Can you work these out from the model? Positions are in its coordinate system, mm. Face numbers are marked on the shaded views. Give positions to 0.01 mm unless a question says otherwise; leave off trailing zeros. Loops run counter-clockwise (first coordinate to the right, second up) from the corner with the lowest first, then second, coordinate; pieces in that order, holes last. Notation, with made-up numbers: (52, -2) -> (86, -2) arc R23 ccw to (86, 17) -> close; hole circle Ø9 at (-27, 9.5). An arc over 180 degrees is marked (long way). Return JSON: item names as keys, results as strings. Group by question number.
Q1. Suppose I cut it at C-C, the plane y = 31. Please give me the cut outline in (x, z).
Q2. I need wall thicknesses on line 1 along Z through (x, y) = (11, 20.5); line 2 along Z through (x, y) = (-0.5, 27); line 3 along X through (y, z) = (44.5, 36). Which ranges of each line are inside material? Lowest first, please. Write a range as [from, to].
Q3. Suppose I cut it at B-B, the plane x = 5. Count the separate pieces of the cut face and the enclosed holes in it, and give its area (3 significant figures).
Q4. Thinking about a two-plate mould opening in X: for the marked faces 1, 2, 3 and 4, which applies, pulls with the +X half, pulls with the -X half, needs draft (parallel to the pull), parting line crosses it, or undercut?
Q5. Suppose I cut it at A-A, the plane y = 4. Please give me the cut outline in (x, z).
```python
from build123d import *

# Parameters (mm, degrees)
SKETCH2_W           = 54.8
SKETCH2_H           = 95
BOSS_EXTRUDE1_DEPTH = 50.8
SKETCH3_R           = 19.05
CUT_EXTRUDE1_DEPTH  = 5
SKETCH4_R           = 14.435817204
SKETCH4_166_R       = 14.435817204


with BuildPart() as part:
    # Sketch2 → Boss-Extrude1 (new body)
    with BuildSketch(Plane(origin=(0, 0, 0), x_dir=(1, 0, 0), z_dir=(0, 1, 0))):
        with Locations((0, -0.795454545)):
            Rectangle(SKETCH2_W, SKETCH2_H)
    extrude(amount=BOSS_EXTRUDE1_DEPTH)

    # Sketch3 → Cut-Extrude1 (cut)
    with BuildSketch(Plane.XZ):
        with Locations(Location((-0.029477, 26.254895545, 0), (0, 0, 270))):
            Circle(SKETCH3_R)
        with Locations(Location((-0.029477, -24.545104455, 0), (0, 0, 90))):
            Circle(SKETCH3_R)
    extrude(amount=-CUT_EXTRUDE1_DEPTH, mode=Mode.SUBTRACT)

    # Sketch4 → section 0 of cut_loft1
    with BuildSketch(Plane(origin=(0, 50.8, 0), x_dir=(1, 0, 0), z_dir=(0, 1, 0)), mode=Mode.PRIVATE) as cut_loft1_s0:
        with Locations((-0.029477, 24.545104455)):
            Circle(SKETCH4_R)
    # loft up to a face of the part (cut_loft1)
    loft([cut_loft1_s0.sketch, Face(Wire([part.edges().sort_by_distance((-13.916329352, 5, -37.585726822))[0]]))], mode=Mode.SUBTRACT)

    # Sketch4<166> → section 0 of cut_loft2
    with BuildSketch(Plane(origin=(0, 50.8, 0), x_dir=(1, 0, 0), z_dir=(0, 1, 0)), mode=Mode.PRIVATE) as cut_loft2_s0:
        with Locations((-0.029477, -26.254895545)):
            Circle(SKETCH4_166_R)
    # loft up to a face of the part (cut_loft2)
    loft([cut_loft2_s0.sketch, Face(Wire([part.edges().sort_by_distance((13.857375352, 5, 39.295517913))[0]]))], mode=Mode.SUBTRACT)


solid = part.part
```
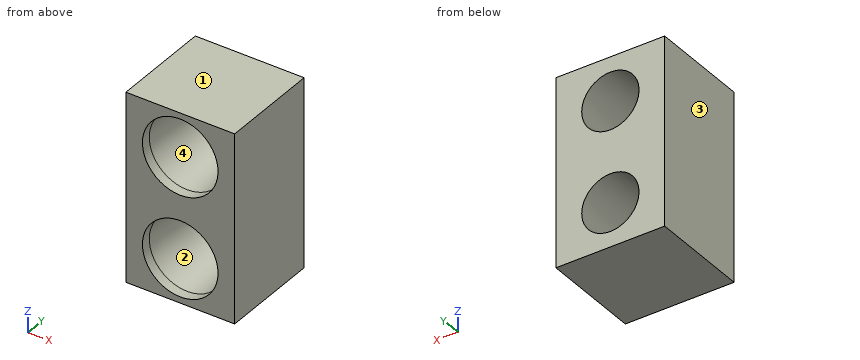
Ans:
{
 "1": {"outline": "(-27.4, -46.7) -> (27.4, -46.7) -> (27.4, 48.3) -> (-27.4, 48.3) -> close; hole circle Ø32.86 at (-0.03, -24.55); hole circle Ø32.86 at (-0.03, 26.25)"},
 "2": {"line 1": "z = [-46.7, -38.12], [-10.97, 12.68], [39.83, 48.3]", "line 2": "z = [-46.7, -41.37], [-7.72, 9.43], [43.08, 48.3]", "line 3": "x = [-27.4, -11.53], [11.47, 27.4]"},
 "3": {"separate pieces": "3", "enclosed holes": "0", "area": "1,530 mm^2"},
 "4": {"face 1": "needs draft", "face 2": "undercut", "face 3": "pulls with the -X half", "face 4": "undercut"},
 "5": {"outline": "(-27.4, -46.7) -> (27.4, -46.7) -> (27.4, 48.3) -> (-27.4, 48.3) -> close; hole circle Ø38.1 at (-0.03, -24.55); hole circle Ø38.1 at (-0.03, 26.25)"}
}
